Input: part model. Units: mm. Frame: model coordinates. A direction names the side the tool comes from. Give positions to 0.01 mm unless a question says otherwise; leave off trailing zeros. Order: outer loops, then holes, each group sorted by start corner. A loop starts at its lowest first (then second) coordinate and runs counter-clockwise, first axis right, second up. Notation, with made-up numbers: M 55,24 L 76,24 A8 cw 76,39 Z; hole C 52.5,50 d6. An arc over 180 degrees is marked long. Use a Markdown table: item, result.
from build123d import *

# Parameters (mm, degrees)
SKETCH1_W           = 20
SKETCH1_H           = 10
SKETCH1_W_2         = 17
SKETCH1_H_2         = 7
BOSS_EXTRUDE1_DEPTH = 220
SKETCH2_R           = 3.25
SKETCH2_R_2         = 2.25
CUT_EXTRUDE1_DEPTH  = 11


with BuildPart() as part:
    # Sketch1 → Boss-Extrude1 (new body)
    with BuildSketch(Plane(origin=(0, 0, 0), x_dir=(0, 0, -1), z_dir=(1, 0, 0))):
        Rectangle(SKETCH1_W, SKETCH1_H)
        Rectangle(SKETCH1_W_2, SKETCH1_H_2, mode=Mode.SUBTRACT)
    extrude(amount=BOSS_EXTRUDE1_DEPTH)

    # Sketch2 → Cut-Extrude1 (cut, through all)
    with BuildSketch(Plane(origin=(0, 5, 0), x_dir=(1, 0, 0), z_dir=(0, 1, 0))):
        with Locations((110, 0)):
            Circle(SKETCH2_R)
        with Locations((150, 0)):
            Circle(SKETCH2_R_2)
    extrude(amount=-CUT_EXTRUDE1_DEPTH, mode=Mode.SUBTRACT)


solid = part.part
1) Reachability of faces 4 (the face through (152.146, 4.26, -0.676)), 5 (the face through (108, 0, -8.5)) from +Z, -Z, +X, -X, +Y, -Y: full face, straight path, thin tool, end or side. Return the list, or none.
Response values:
| item | result |
|---|---|
| face 4 | +Y, -Y |
| face 5 | +X, -X |
2) Material intervals for line 1 (X direction, y = 4.05, z = 0); line 2 (Z direction, x = 208.5, y = 0.75); line 3 (Y direction, x = 130, z = 1.75), sorted ascending. Write a range as from..to.
Response values:
| item | result |
|---|---|
| line 1 | x = 0..106.75, 113.25..147.75, 152.25..220 |
| line 2 | z = -10..-8.5, 8.5..10 |
| line 3 | y = -5..-3.5, 3.5..5 |
3) Cut plane C-C on y = 1. Return loops of the section in (x, z), and give its area (3 significant figures).
Response values:
| item | result |
|---|---|
| outline | M 0,-10 L 220,-10 L 220,-8.5 L 0,-8.5 Z; M 0,8.5 L 220,8.5 L 220,10 L 0,10 Z |
| area | 660 mm² |
4) Cut plane B-B on x = 54. Return loops of the section in (y, z).
Response values:
| item | result |
|---|---|
| outline | M -5,-10 L 5,-10 L 5,10 L -5,10 Z; hole M -3.5,-8.5 L 3.5,-8.5 L 3.5,8.5 L -3.5,8.5 Z |
5) Mould query, pull axis Y, two halves, no side actions, for faces 1 (the face through (108, 0, 8.5)), 2 (the face through (220, -4, 0)), 3 (the face through (108, -5, -4)). Classes: released by +Y, released by -Y, zero draft, split by the parting line, or undercut.
Response values:
| item | result |
|---|---|
| face 1 | undercut |
| face 2 | zero draft |
| face 3 | released by -Y |
6) Cut plane D-D on x = 110. Return loops of the section in (y, z).
Response values:
| item | result |
|---|---|
| outline | M -5,-10 L 5,-10 L 5,-3.25 L 3.5,-3.25 L 3.5,-8.5 L -3.5,-8.5 L -3.5,-3.25 L -5,-3.25 Z; M -5,3.25 L -3.5,3.25 L -3.5,8.5 L 3.5,8.5 L 3.5,3.25 L 5,3.25 L 5,10 L -5,10 Z |
7) Cut plane A-A on z = -6.25. Return loops of the section in (x, y), and give its area (3 significant figures).
Response values:
| item | result |
|---|---|
| outline | M 0,-5 L 220,-5 L 220,-3.5 L 0,-3.5 Z; M 0,3.5 L 220,3.5 L 220,5 L 0,5 Z |
| area | 660 mm² |
